Check sheet for the drawn part. Datum: minimum x, y, z corner. Units: mm. A direction names the side the tool comes from. Coordinates: 2 decimals unless noted, no trailing zeros. Write each loop counter-clockwise with the first axis right and the second up, starting at its lowest first coordinate (ties: lowest second). Pieces come first, ordered by that corner, then holes. Notation, with made-up numbers: (56.25, 9) -> (80.25, 9) arc R11 cw to (80.25, 28) -> close; hole circle Ø5 at (-30.75, 84). An arc over 180 degrees is marked (long way). Answer in a Markdown table with one row per item.
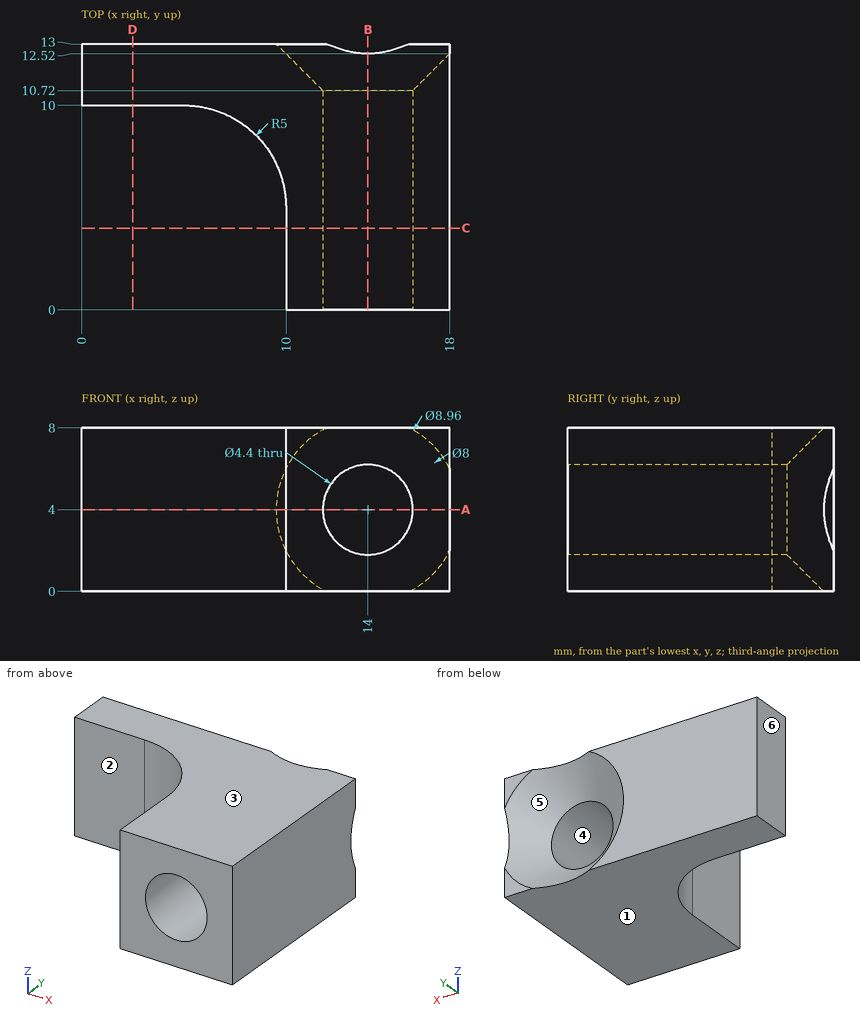
1. Go/stop test with flat-tipped pins: pin 1 (1.5 mm diameter, centred on x = 3, z = 3.5, fed in from -Y); pin 2 (2.5 mm diameter, centred on x = 14, z = 4, fed in from -Y); pin 3 (3 mm diameter, centred on x = 8, y = 8, fed in from +Z); pin 4 (1 mm diameter, centred on y = 2, z = 2.5, fed in from -X). Record where each tip stops, or that it passes through.
Findings below:
| item | result |
|---|---|
| pin 1 | stops at y = 10 |
| pin 2 | passes through |
| pin 3 | stops at z = 8 |
| pin 4 | stops at x = 10 |
2. Release check for a two-part mould opening along Z. For the marked faces 3, 4, 5 and 6 record: released by +Z, released by -Z, zero draft, split by the parting line, or undercut.
Findings below:
| item | result |
|---|---|
| face 3 | released by +Z |
| face 4 | undercut |
| face 5 | undercut |
| face 6 | zero draft |
3. Sectioned sample at B-B, the plane x = 14. Record the cut outline in (y, z).
Findings below:
| item | result |
|---|---|
| outline | (0, 0) -> (12.52, 0) -> (10.72, 1.8) -> (0, 1.8) -> close; (0, 6.2) -> (10.72, 6.2) -> (12.52, 8) -> (0, 8) -> close |
4. Sectioned sample at D-D, the plane x = 2.5. Record the cut outline in (y, z).
Findings below:
| item | result |
|---|---|
| outline | (10, 0) -> (13, 0) -> (13, 8) -> (10, 8) -> close |
5. Sectioned sample at A-A, the plane z = 4. Record the cut outline in (x, y), and give its area (3 significant figures).
Findings below:
| item | result |
|---|---|
| outline | (0, 10) -> (5, 10) arc R5 cw to (10, 5) -> (10, 0) -> (11.8, 0) -> (11.8, 10.72) -> (9.52, 13) -> (0, 13) -> close; (16.2, 0) -> (18, 0) -> (18, 12.52) -> (16.2, 10.72) -> close |
| area | 77.1 mm² |
6. Material ranges on probe 1 along Z at (x, y) = (14, 7); probe 2 along Y at (x, z) = (4.5, 7.5); probe 3 along Z at (x, y) = (14.75, 12.25), recorded low to high. Write a range as from..to.
Findings below:
| item | result |
|---|---|
| probe 1 | z = 0..1.8, 6.2..8 |
| probe 2 | y = 10..13 |
| probe 3 | z = 0..0.35, 7.65..8 |
7. Sectioned sample at C-C, the plane y = 4. Record the cut outline in (x, z), and give its area (3 significant figures).
Findings below:
| item | result |
|---|---|
| outline | (10, 0) -> (18, 0) -> (18, 8) -> (10, 8) -> close; hole circle Ø4.4 at (14, 4) |
| area | 48.8 mm² |
8. Access from +Z, -Z, +X, -X, +Y, -Y to the whole of each face (thin tool, end or side, straight path). Record for the marked faces 1 and 2.
Findings below:
| item | result |
|---|---|
| face 1 | -Z, +X, -X, +Y, -Y |
| face 2 | +Z, -Z, -X, -Y |
